Geometry check sheet. Reference: the model listing, model coordinates, mm. Round coordinates to 2 decimals unless told otherwise and drop trailing zeros. Write each loop counter-clockwise with the first axis right and the second up, starting at its lowest first coordinate (ties: lowest second). Pieces come first, ordered by that corner, then holes.
Item 1: Cross-section at D-D (x = -31.75). Enter the section's corners in (y, z), then the cut area to 3 significant figures.
Item 2: Scan lines: probe 1 along X at (y, z) = (4, -21); probe 2 along X at (y, z) = (5.75, -0.5); probe 3 along Z at (x, y) = (0, 3.5). Record each from-to range of solid material in increasing order.
Item 3: Draft check along Z on faces 1 (the face through (146.05, 3, 16)), 2 (the face through (-33.274, 3.131, 57.963)), 3 (the face through (52, 3, 67.733)), 4 (the face through (-2.93, 3.13, 39.5)). Enter one of: pulls with the +Z half, pulls with the -Z half, needs draft (parallel to the pull), parting line crosses it, or undercut.
Item 4: Depth check by flat-ended pin: P1, Ø6, axis at x = -31.75, z = 55.03, coming from the -Y side. Enter the tip coordinate at first touch or a pass-through.
Item 5: Cross-section at A-A (x = 0). Enter the section's corners in (y, z).
Item 6: Cross-section at B-B (z = 0). Enter the section's corners in (x, y).
Item 7: Cross-section at C-C (y = 1.5). State how many separate pieces and enclosed holes the cut face has, then the cut area to 3 significant figures.
Autodesk Inventor part; units mm, degrees
ref_plane "YZ Plane" through (0, 0, 0) normal (1, 0, 0) x (0, 1, 0)
ref_plane "XZ Plane" through (0, 0, 0) normal (0, 1, 0) x (-1, 0, 0)
ref_plane "XY Plane" through (0, 0, 0) normal (0, 0, 1) x (1, 0, 0)
sketch "Sketch1" plane through (0, 0, 0) normal (0, 1, 0) x (-1, 0, 0)
  circle A0 centre (0, 0) radius 6.35
  line L0 (0, 0) -> (0, 25.4) construction
  line L1 (0, 0) -> (-101.6, 0) construction
  line L2 (44.45, -33.8667) -> (-146.05, -33.8667)
  line L3 (-146.05, -33.8667) -> (-146.05, 67.7333)
  line L4 (-146.05, 67.7333) -> (44.45, 67.7333)
  line L5 (44.45, 67.7333) -> (44.45, -33.8667)
  circle A1 centre (31.75, -21.1667) radius 3.302
  circle A2 centre (-133.35, -21.1667) radius 3.302
  circle A3 centre (-133.35, 55.0333) radius 3.302
  circle A4 centre (31.75, 55.0333) radius 3.302
  circle A5 centre (-33.8667, 0) radius 6.35
  circle A6 centre (-67.7333, 0) radius 6.35
  circle A7 centre (-101.6, 0) radius 6.35
  circle A8 centre (0, 33.8667) radius 6.35
  circle A9 centre (-33.8667, 33.8667) radius 6.35
  circle A10 centre (-67.7333, 33.8667) radius 6.35
  circle A11 centre (-101.6, 33.8667) radius 6.35
  dimension "d0" = 12.7
  dimension "d15" = 6.604
  dimension "d16" = 12.7
  dimension "d17" = 12.7
  dimension "d18" = 6.604
  dimension "d19" = 12.7
  dimension "d20" = 6.604
  dimension "d21" = 12.7
  dimension "d22" = 6.604
  dimension "d25" = 101.6
  dimension "d26" = 33.8667
  dimension "d27" = 12.7
  dimension "d28" = 12.7
  dimension "d29" = 12.7
  dimension "d30" = 44.45
  dimension "d31" = 190.5
  dimension "d34" = 33.8667
  dimension "d37" = 33.8667
extrude "Extrusion2" add sketch "Sketch1" along normal blind 6.35
equation "\"d37\" = 0.333333 * d25"
properties part number "SequenceMachine_VialPlate"
Resolved:
1. outline: (0, -33.87) - (6.35, -33.87) - (6.35, -24.47) - (0, -24.47) - close; (0, -17.86) - (6.35, -17.86) - (6.35, 51.73) - (0, 51.73) - close; (0, 58.34) - (6.35, 58.34) - (6.35, 67.73) - (0, 67.73) - close
1. area: 561 mm2
2. probe 1: x = -44.45 to -35.05, -28.45 to 130.05, 136.65 to 146.05
2. probe 2: x = -44.45 to -6.33, 6.33 to 27.54, 40.2 to 61.4, 74.06 to 95.27, 107.93 to 146.05
2. probe 3: z = -33.87 to -6.35, 6.35 to 27.52, 40.22 to 67.73
3. face 1: needs draft
3. face 2: undercut
3. face 3: pulls with the +Z half
3. face 4: undercut
4. P1: passes through
5. outline: (0, -33.87) - (6.35, -33.87) - (6.35, -6.35) - (0, -6.35) - close; (0, 6.35) - (6.35, 6.35) - (6.35, 27.52) - (0, 27.52) - close; (0, 40.22) - (6.35, 40.22) - (6.35, 67.73) - (0, 67.73) - close
6. outline: (-44.45, 0) - (-6.35, 0) - (-6.35, 6.35) - (-44.45, 6.35) - close; (6.35, 0) - (27.52, 0) - (27.52, 6.35) - (6.35, 6.35) - close; (40.22, 0) - (61.38, 0) - (61.38, 6.35) - (40.22, 6.35) - close; (74.08, 0) - (95.25, 0) - (95.25, 6.35) - (74.08, 6.35) - close; (107.95, 0) - (146.05, 0) - (146.05, 6.35) - (107.95, 6.35) - close
7. separate pieces: 1
7. enclosed holes: 12
7. area: 18,200 mm2
